Input: part model. Units: mm. Frame: model coordinates. Face numbers are marked on the shaded views. A direction names the side the tool comes from. Coordinates: 2 decimals unless noted, no trailing zeros. Order: outer loops, then holes, each group sorted by start corner. A loop starts at its lowest first (then second) coordinate and runs counter-clockwise, first axis right, second up.
from build123d import *

# Parameters (mm, degrees)
SKETCH2_R           = 30
SKETCH2_R_2         = 105
SKETCH2_R_3         = 28.090856429
SKETCH2_R_4         = 15
BOSS_EXTRUDE2_DEPTH = 50
SKETCH5_R           = 30
CUT_EXTRUDE1_DEPTH  = 10
CHAMFER2_SIZE       = 10
BOSS_EXTRUDE3_START = 100
SKETCH6_R           = 145
SKETCH6_R_2         = 105
BOSS_EXTRUDE3_DEPTH = 100
CUT_EXTRUDE2_START  = -10
SKETCH9_R           = 30
SKETCH9_R_2         = 15
CUT_EXTRUDE2_DEPTH  = 10
SWEEP3_OUTLINE_R    = 145
SWEEP3_OUTLINE_R_2  = 105
SWEEP3_ANGLE        = 90
SKETCH12_R          = 145
SKETCH12_R_2        = 105
BOSS_EXTRUDE5_DEPTH = 100
BOSS_EXTRUDE6_DEPTH = 50
SKETCH14_R          = 105
CUT_EXTRUDE5_DEPTH  = 50
SKETCH17_R          = 30
SKETCH17_R_2        = 15
CUT_EXTRUDE6_DEPTH  = 10
SKETCH18_R          = 15
SKETCH18_R_2        = 14.143688161
CUT_EXTRUDE7_DEPTH  = 100
CHAMFER3_SIZE       = 10


# Read off the part's stored shape, not the designer's step: Sweep3
with BuildPart() as part:
    # Sketch2 → Boss-Extrude2 (new body)
    # profile 1 of 5: a face of its own
    with BuildSketch(Plane(origin=(0, 0, 0), x_dir=(1, 0, 0), z_dir=(0, 1, 0))):
        with BuildLine():
            Line((-180, -130), (-180, -160))
            ThreePointArc((-180, -160), (-174.142135624, -174.142135624), (-160, -180))
            Line((-160, -180), (160, -180))
            ThreePointArc((160, -180), (174.142135624, -174.142135624), (180, -160))
            Line((180, -160), (180, 160))
            ThreePointArc((180, 160), (174.142135624, 174.142135624), (160, 180))
            Line((160, 180), (-160, 180))
            ThreePointArc((-160, 180), (-174.142135624, 174.142135624), (-180, 160))
            Line((-180, 160), (-180, -130))
        make_face()
        with Locations((-130, -130)):
            Circle(SKETCH2_R, mode=Mode.SUBTRACT)
        with Locations((130, -130)):
            Circle(SKETCH2_R, mode=Mode.SUBTRACT)
        with Locations((-130, 130)):
            Circle(SKETCH2_R, mode=Mode.SUBTRACT)
        with Locations(Location((0, 0, 0), (0, 0, 270))):
            Circle(SKETCH2_R_2, mode=Mode.SUBTRACT)
        with Locations((130, 130)):
            Circle(SKETCH2_R_3, mode=Mode.SUBTRACT)
    # profile 2 of 5: a face of its own
    with BuildSketch(Plane(origin=(0, 0, 0), x_dir=(1, 0, 0), z_dir=(0, 1, 0))):
        with Locations((-130, 130)):
            Circle(SKETCH2_R)
        with Locations(Location((-130, 130, 0), (0, 0, 270))):
            Circle(SKETCH2_R_4, mode=Mode.SUBTRACT)
    # profile 3 of 5: a face of its own
    with BuildSketch(Plane(origin=(0, 0, 0), x_dir=(1, 0, 0), z_dir=(0, 1, 0))):
        with Locations((130, 130)):
            Circle(SKETCH2_R_3)
        with Locations(Location((130, 130, 0), (0, 0, 270))):
            Circle(SKETCH2_R_4, mode=Mode.SUBTRACT)
    # profile 4 of 5: a face of its own
    with BuildSketch(Plane(origin=(0, 0, 0), x_dir=(1, 0, 0), z_dir=(0, 1, 0))):
        with Locations((-130, -130)):
            Circle(SKETCH2_R)
        with Locations(Location((-130, -130, 0), (0, 0, 270))):
            Circle(SKETCH2_R_4, mode=Mode.SUBTRACT)
    # profile 5 of 5: a face of its own
    with BuildSketch(Plane(origin=(0, 0, 0), x_dir=(1, 0, 0), z_dir=(0, 1, 0))):
        with Locations((130, -130)):
            Circle(SKETCH2_R)
        with Locations(Location((130, -130, 0), (0, 0, 270))):
            Circle(SKETCH2_R_4, mode=Mode.SUBTRACT)
    extrude(amount=BOSS_EXTRUDE2_DEPTH)

    # Sketch5 → Cut-Extrude1 (cut)
    with BuildSketch(Plane(origin=(0, 50, 0), x_dir=(1, 0, 0), z_dir=(0, 1, 0))):
        with Locations(Location((-130, 130, 0), (0, 0, 270))):
            Circle(SKETCH5_R)
        with Locations(Location((130, 130, 0), (0, 0, 270))):
            Circle(SKETCH5_R)
        with Locations(Location((-130, -130, 0), (0, 0, 270))):
            Circle(SKETCH5_R)
    extrude(amount=-CUT_EXTRUDE1_DEPTH, mode=Mode.SUBTRACT)

    # Chamfer2
    chamfer2_edges = [part.edges().sort_by_distance(p)[0] for p in [
        (0, 50, -105),
    ]]
    chamfer(chamfer2_edges, length=CHAMFER2_SIZE)

    # Sketch6 → Boss-Extrude3 (add)
    with BuildSketch(Plane.XZ.offset(BOSS_EXTRUDE3_START)):
        with Locations(Location((0, 0, 0), (0, 0, 90))):
            Circle(SKETCH6_R)
        with Locations(Location((0, 0, 0), (0, 0, 270))):
            Circle(SKETCH6_R_2, mode=Mode.SUBTRACT)
    extrude(amount=-BOSS_EXTRUDE3_DEPTH)

    # Sketch9 → Cut-Extrude2 (cut)
    with BuildSketch(Plane(origin=(0, 50, 0), x_dir=(1, 0, 0), z_dir=(0, 1, 0)).offset(CUT_EXTRUDE2_START)):
        with Locations(Location((130, -130, 0), (0, 0, 270))):
            Circle(SKETCH9_R)
        with Locations(Location((130, -130, 0), (0, 0, 270))):
            Circle(SKETCH9_R_2, mode=Mode.SUBTRACT)
    extrude(amount=CUT_EXTRUDE2_DEPTH, mode=Mode.SUBTRACT)

    # Sweep3 outline → Sweep3 (revolve)
    with BuildSketch(Plane(origin=(260, -100, 0), x_dir=(-1, 0, 0), z_dir=(0, 1, 0))):
        with Locations((260, 0)):
            Circle(SWEEP3_OUTLINE_R)
        with Locations((260, 0)):
            Circle(SWEEP3_OUTLINE_R_2, mode=Mode.SUBTRACT)
    revolve(axis=Axis((260, -100, 0), (0, 0, 1)), revolution_arc=SWEEP3_ANGLE)

    # Sketch12 → Boss-Extrude5 (add)
    with BuildSketch(Plane(origin=(260, 0, 0), x_dir=(0, 0, -1), z_dir=(1, 0, 0))):
        with Locations(Location((0, -360, 0), (0, 0, 270))):
            Circle(SKETCH12_R)
        with Locations(Location((0, -360, 0), (0, 0, 270))):
            Circle(SKETCH12_R_2, mode=Mode.SUBTRACT)
    extrude(amount=BOSS_EXTRUDE5_DEPTH)

    # Sketch13 → Boss-Extrude6 (add)
    with BuildSketch(Plane(origin=(360, 0, 0), x_dir=(0, 0, -1), z_dir=(1, 0, 0))):
        with BuildLine():
            Line((-170, -540), (170, -540))
            ThreePointArc((170, -540), (177.071067812, -537.071067812), (180, -530))
            Line((180, -530), (180, -190))
            ThreePointArc((180, -190), (177.071067812, -182.928932188), (170, -180))
            Line((170, -180), (-170, -180))
            ThreePointArc((-170, -180), (-177.071067812, -182.928932188), (-180, -190))
            Line((-180, -190), (-180, -530))
            ThreePointArc((-180, -530), (-177.071067812, -537.071067812), (-170, -540))
        make_face()
    extrude(amount=BOSS_EXTRUDE6_DEPTH)

    # Sketch14 → Cut-Extrude5 (cut)
    with BuildSketch(Plane(origin=(410, 0, 0), x_dir=(0, 0, -1), z_dir=(1, 0, 0))):
        with Locations(Location((0, -369.029004143, 0), (0, 0, 90))):
            Circle(SKETCH14_R)
    extrude(amount=-CUT_EXTRUDE5_DEPTH, mode=Mode.SUBTRACT)

    # Sketch17 → Cut-Extrude6 (cut)
    # profile 1 of 4: a face of its own
    with BuildSketch(Plane(origin=(410, 0, 0), x_dir=(0, 0, -1), z_dir=(1, 0, 0))):
        with Locations(Location((-130, -230, 0), (0, 0, 90))):
            Circle(SKETCH17_R)
        with Locations(Location((-130, -230, 0), (0, 0, 90))):
            Circle(SKETCH17_R_2, mode=Mode.SUBTRACT)
    # profile 2 of 4: a face of its own
    with BuildSketch(Plane(origin=(410, 0, 0), x_dir=(0, 0, -1), z_dir=(1, 0, 0))):
        with Locations(Location((-130, -490, 0), (0, 0, 90))):
            Circle(SKETCH17_R)
        with Locations(Location((-130, -490, 0), (0, 0, 90))):
            Circle(SKETCH17_R_2, mode=Mode.SUBTRACT)
    # profile 3 of 4: a face of its own
    with BuildSketch(Plane(origin=(410, 0, 0), x_dir=(0, 0, -1), z_dir=(1, 0, 0))):
        with Locations(Location((130, -490, 0), (0, 0, 90))):
            Circle(SKETCH17_R)
        with Locations(Location((130, -490, 0), (0, 0, 90))):
            Circle(SKETCH17_R_2, mode=Mode.SUBTRACT)
    # profile 4 of 4: a face of its own
    with BuildSketch(Plane(origin=(410, 0, 0), x_dir=(0, 0, -1), z_dir=(1, 0, 0))):
        with Locations(Location((130, -230, 0), (0, 0, 90))):
            Circle(SKETCH17_R)
        with Locations(Location((130, -230, 0), (0, 0, 90))):
            Circle(SKETCH17_R_2, mode=Mode.SUBTRACT)
    extrude(amount=-CUT_EXTRUDE6_DEPTH, mode=Mode.SUBTRACT)

    # Sketch18 → Cut-Extrude7 (cut)
    with BuildSketch(Plane(origin=(410, 0, 0), x_dir=(0, 0, -1), z_dir=(1, 0, 0))):
        with Locations(Location((-130, -230, 0), (0, 0, 90))):
            Circle(SKETCH18_R)
        with Locations(Location((130, -230, 0), (0, 0, 90))):
            Circle(SKETCH18_R)
        with Locations(Location((-130, -490, 0), (0, 0, 90))):
            Circle(SKETCH18_R)
        with Locations(Location((130, -490, 0), (0, 0, 90))):
            Circle(SKETCH18_R_2)
    extrude(amount=-CUT_EXTRUDE7_DEPTH, mode=Mode.SUBTRACT)

    # Chamfer3
    chamfer3_edges = [part.edges().sort_by_distance(p)[0] for p in [
        (410, -474.029004143, 0),
    ]]
    chamfer(chamfer3_edges, length=CHAMFER3_SIZE)


solid = part.part
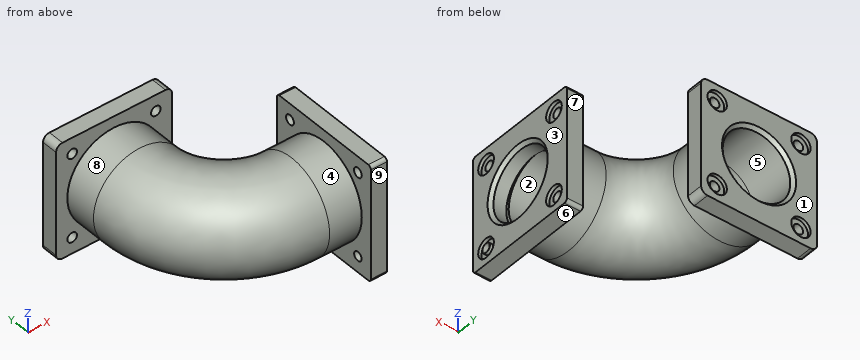
Item 1: Cut plane A-A on x = 349.5. Return loops of the section in (y, z), then the cut area to 3 significant figures.
Response values:
outline: circle Ø290 at (-360, 0); hole circle Ø210 at (-360, 0)
area: 31,400 mm2
Item 2: Access query for the marked faces 5, 6, 7, 8 and 9. Directions: +Z, -Z, +X, -X, +Y, -Y. A direction counts if a zero-diameter tool reaches every point of the face in a straight line with its end or side. Return the directions, or none.
Response values:
face 5: +Y
face 6: -Z, +X, -X, +Y, -Y
face 7: +Z, -Z, +X, +Y
face 8: none
face 9: +Z, -Z, +X, -X, -Y
Item 3: Cut plane C-C on z = -130. Count the separate pieces of the cut face and the enclosed holes in it, then the cut area to 3 significant figures.
Response values:
separate pieces: 5
enclosed holes: 0
area: 107,000 mm2
Item 4: Draft query along X for the marked faces 1, 2, 3 and 4. Return one class per face: pulls with the +X half, pulls with the -X half, needs draft (parallel to the pull), parting line crosses it, or undercut.
Response values:
face 1: needs draft
face 2: undercut
face 3: pulls with the +X half
face 4: undercut
Item 5: Cut plane B-B on y = -64. Return loops of the section in (x, z), then the cut area to 3 significant figures.
Response values:
outline: circle Ø290 at (0, 0); hole circle Ø210 at (0, 0)
area: 31,400 mm2
Item 6: Pin query (flat end, axial travel): pin 1 Ø2 at (x, z) = (76, 73.5) entering from -Y; pin 2 Ø8 at (x, y) = (23.5, -213) entering from +Z; pin 3 Ø3 at (y, z) = (-94.5, -69.5) entering from -X. Return the tip coordinate at first contact, or that it passes through.
Response values:
pin 1: stops at y = -439.03
pin 2: stops at z = 145
pin 3: stops at x = -128.07
Item 7: Ray query, probe 1 along X at (y, z) = (19, -130); probe 2 along X at (y, z) = (45.25, 130); probe 3 along Y at (x, z) = (159.5, 78.5). Return the intervals inside material, ascending.
Response values:
probe 1: x = -180 to -145, -115 to 115, 145 to 180
probe 2: x = -180 to -160, -100 to 100, 160 to 180
probe 3: y = -468.45 to -414.04, -261.56 to -194.7, 0 to 50
